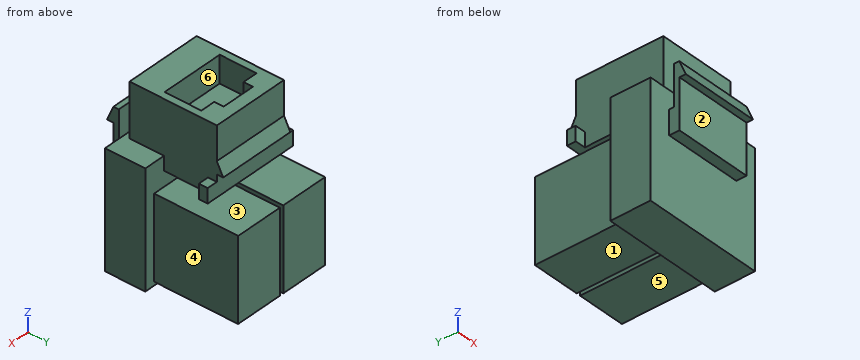
from build123d import *

# Parameters (mm, degrees)
ESBO_O1_W                = 14.5
ESBO_O1_H                = 16.25
RESSALTO_EXTRUS_O1_DEPTH = 12.5
RESSALTO_EXTRUS_O2_DEPTH = 14.5
ESBO_O3_W                = 18.45
ESBO_O3_H                = 2.7
RESSALTO_EXTRUS_O3_DEPTH = 1.65
CORTE_EXTRUS_O1_DEPTH    = 5
RESSALTO_EXTRUS_O4_START = -9.9
ESBO_O5_W                = 22.55
ESBO_O5_H                = 7.5
RESSALTO_EXTRUS_O4_DEPTH = 21.4
ESBO_O6_W                = 9
ESBO_O6_H                = 15.3
RESSALTO_EXTRUS_O5_DEPTH = 15.65
RESSALTO_EXTRUS_O6_DEPTH = 14.5
RESSALTO_EXTRUS_O7_DEPTH = 14.5


with BuildPart() as part:
    # Esboço1 → Ressalto-extrusão1 (new body)
    with BuildSketch(Plane.XY):
        Rectangle(ESBO_O1_W, ESBO_O1_H)
    extrude(amount=RESSALTO_EXTRUS_O1_DEPTH)

    # Esboço2 → Ressalto-extrusão2 (add)
    with BuildSketch(Plane.ZY.offset(7.25)):
        Polygon((6.3, 8.125), (4, 9.305), (4, 8.125), align=None)
    extrude(amount=-RESSALTO_EXTRUS_O2_DEPTH)

    # Esboço3 → Ressalto-extrusão3 (add)
    with BuildSketch(Plane(origin=(0, 8.125, 0), x_dir=(1, 0, 0), z_dir=(0, 1, 0))):
        with Locations((0, -1.35)):
            Rectangle(ESBO_O3_W, ESBO_O3_H)
    extrude(amount=-RESSALTO_EXTRUS_O3_DEPTH)

    # Esboço4 → Corte-extrusão1 (cut)
    with BuildSketch(Plane.XY.offset(12.5)):
        Polygon((-5.95, 4.125), (-3.175, 4.125), (-3.175, 5.875), (3.175, 5.875), (3.175, 4.125), (5.95, 4.125), (5.95, -2.725), (-5.95, -2.725), align=None)
    extrude(amount=-CORTE_EXTRUS_O1_DEPTH, mode=Mode.SUBTRACT)

    # Esboço5 → Ressalto-extrusão4 (add)
    with BuildSketch(Plane.XY.offset(12.5).offset(RESSALTO_EXTRUS_O4_START)):
        with Locations((0, -5.475)):
            Rectangle(ESBO_O5_W, ESBO_O5_H)
    extrude(amount=-RESSALTO_EXTRUS_O4_DEPTH)

    # Esboço6 → Ressalto-extrusão5 (add)
    with BuildSketch(Plane(origin=(0, -1.725, 0), x_dir=(1, 0, 0), z_dir=(0, 1, 0))):
        with Locations((-4.875, 10.45)):
            Rectangle(ESBO_O6_W, ESBO_O6_H)
        with Locations((4.875, 10.45)):
            Rectangle(ESBO_O6_W, ESBO_O6_H)
    extrude(amount=RESSALTO_EXTRUS_O5_DEPTH)

    # Esboço7 → Ressalto-extrusão6 (add)
    with BuildSketch(Plane.ZY.offset(7.25)):
        Polygon((-5.28, -9.225), (-5.28, -11.125), (6.72, -11.125), (6.72, -10.125), (-0.78, -10.125), (-0.78, -9.225), align=None)
    extrude(amount=-RESSALTO_EXTRUS_O6_DEPTH)

    # Esboço8 → Ressalto-extrusão7 (add)
    with BuildSketch(Plane.ZY.offset(7.25)):
        Polygon((6.72, -11.125), (3.92, -12.325), (3.92, -11.125), align=None)
    extrude(amount=-RESSALTO_EXTRUS_O7_DEPTH)


solid = part.part
Build history of the part. All positions in model axes, mm. Face numbers are marked on the shaded views. A direction names the side the tool comes from. Give positions to 0.01 mm unless a question says otherwise; leave off trailing zeros. Order: outer loops, then holes, each group sorted by start corner. A loop starts at its lowest first (then second) coordinate and runs counter-clockwise, first axis right, second up. Notation, with made-up numbers: M 38,80.25 L 81,80.25 A16 ccw 81,111.25 Z; hole C 64.25,30 d9. An arc over 180 degrees is marked long. Use one line per item in the form item = value.
Q1. Slice it at C-C, the plane z = 9. Write the cut outline in (x, y) (3 decimals).
Conclusion:
outline = M -7.25,-8.125 L 7.25,-8.125 L 7.25,8.125 L -7.25,8.125 Z; hole M -5.95,-2.725 L 5.95,-2.725 L 5.95,4.125 L 3.175,4.125 L 3.175,5.875 L -3.175,5.875 L -3.175,4.125 L -5.95,4.125 Z
Q2. Slice it at A-A, the plane z = 3.5. Write the cut outline in (x, y) (3 decimals).
Conclusion:
outline = M -7.25,-11.125 L 7.25,-11.125 L 7.25,-10.125 L -7.25,-10.125 Z; M -7.25,-8.125 L 7.25,-8.125 L 7.25,8.125 L -7.25,8.125 Z
Q3. Slice it at D-D, the plane x = -5. Write the cut outline in (y, z) (3 decimals), and give its area (3 significant figures).
Conclusion:
outline = M -12.325,3.92 L -11.125,3.92 L -11.125,-5.28 L -9.225,-5.28 L -9.225,-18.8 L -1.725,-18.8 L -1.725,-18.1 L 13.925,-18.1 L 13.925,-2.8 L -1.725,-2.8 L -1.725,0 L 8.125,0 L 8.125,4 L 9.305,4 L 8.125,6.3 L 8.125,12.5 L 4.125,12.5 L 4.125,7.5 L -2.725,7.5 L -2.725,12.5 L -8.125,12.5 L -8.125,2.6 L -9.225,2.6 L -9.225,-0.78 L -10.125,-0.78 L -10.125,6.72 L -11.125,6.72 Z
area = 571 mm2
Q4. Pin check, flat tips, straight feed: P1, Ø3, axis at x = -1, y = 8.5, coming from the -Z side; P2, Ø8, axis at x = 7, z = -12.5, coming from the -Y side (3 decimals); P3, Ø3, axis at x = 2.5, z = 9.5, coming from the +Y side (3 decimals). Stop position of each tip, or through.
Conclusion:
P1 = -18.1
P2 = -9.225
P3 = 8.125
Q5. Wall check: probe 1 along X at (y, z) = (-0.25, -9) (3 decimals); probe 2 along Y at (x, z) = (-1.5, 9) (3 decimals); probe 3 along Z at (x, y) = (2.75, 2.25). Give the ranges that are in metal, low to high.
Conclusion:
probe_1 = -9.375 to -0.375, 0.375 to 9.375
probe_2 = -8.125 to -2.725, 5.875 to 8.125
probe_3 = -18.1 to -2.8, 0 to 7.5
Q6. Pull direction Z, two halves, no side cores. Call the marked faces 1, 2 and 3: released by +Z, released by -Z, zero draft, split by the parting line, or undercut.
Conclusion:
face_1 = released by -Z
face_2 = zero draft
face_3 = undercut
Q7. Slice it at B-B, the plane y = 11. Write the cut outline in (x, z) (3 decimals).
Conclusion:
outline = M -9.375,-18.1 L -0.375,-18.1 L -0.375,-2.8 L -9.375,-2.8 Z; M 0.375,-18.1 L 9.375,-18.1 L 9.375,-2.8 L 0.375,-2.8 Z
Q8. Which spindle directions (+Z, -Z, +X, -X, +Y, -Y) get a long thin tool onto all of the face, cutting with end or side? Do the marked faces 4, 5 and 6. Say none if no direction does.
Conclusion:
face_4 = +Z, -Z, +X, +Y
face_5 = -Z, +X, -X, +Y
face_6 = +Z
